Geometry check sheet. Reference: the model listing, model coordinates, mm. Round coordinates to 2 decimals unless told otherwise and drop trailing zeros. Order: outer loops, then holes, each group sorted by start corner. A loop starts at its lowest first (then second) coordinate and runs counter-clockwise, first axis right, second up.
```python
from build123d import *

# Parameters (mm, degrees)
F0_W          = 2.54
F0_H          = 2.54
F1_DEPTH      = 2.5
F2_SIZE       = 0.25
F3_W          = 0.7
F3_H          = 0.7
F4_DEPTH      = 2.7
F4_DEPTH_BACK = 8.9
F5_SIZE       = 0.1


with BuildPart() as f1:
    # F0 (on Top) → F1 (new body)
    with BuildSketch(Plane.XY):
        Rectangle(F0_W, F0_H)
    extrude(amount=F1_DEPTH)

    # F2
    f2_edges = [f1.edges().sort_by_distance(p)[0] for p in [
        (-1.27, -1.27, 1.25),
        (1.27, -1.27, 1.25),
        (1.27, 1.27, 1.25),
        (-1.27, 1.27, 1.25),
        (0, 1.27, 2.5),
        (1.27, 0, 2.5),
        (0, -1.27, 2.5),
        (-1.27, 0, 2.5),
        (1.27, 0, 0),
        (0, -1.27, 0),
        (-1.27, 0, 0),
        (0, 1.27, 0),
    ]]
    chamfer(f2_edges, length=F2_SIZE)

    # F3 (on face) → F4 (join, two sides)
    with BuildSketch(Plane.XY.offset(2.5)) as f4_sk:
        Rectangle(F3_W, F3_H)
    extrude(amount=F4_DEPTH)
    extrude(f4_sk.sketch, amount=-F4_DEPTH_BACK)

    # F5
    f5_edges = [f1.edges().sort_by_distance(p)[0] for p in [
        (0.35, 0, 5.2),
        (0, 0.35, 5.2),
        (-0.35, 0, 5.2),
        (0, -0.35, 5.2),
        (0.35, 0, -6.4),
        (0, -0.35, -6.4),
        (-0.35, 0, -6.4),
        (0, 0.35, -6.4),
    ]]
    chamfer(f5_edges, length=F5_SIZE)


solid = f1.part
```
(1) Depth check by flat-ended pin: P1, Ø0.8, axis at x = 0, z = -3, coming from the +Y side; P2, Ø0.8, axis at y = 0, z = 4, coming from the +X side; P3, Ø0.8, axis at y = 0, z = -4, coming from the -X side. Enter the tip coordinate at first touch or a pass-through.
Returned:
P1: stops at y = 0.35
P2: stops at x = 0.35
P3: stops at x = -0.35
(2) Sectioned sample at C-C, the plane z = 1.75. Record the cut outline in (x, y), and give its area (3 significant figures).
Returned:
outline: (-1.27, -1.02) - (-1.02, -1.27) - (1.02, -1.27) - (1.27, -1.02) - (1.27, 1.02) - (1.02, 1.27) - (-1.02, 1.27) - (-1.27, 1.02) - close
area: 6.33 mm2
(3) Sectioned sample at B-B, the plane x = -0.75. Record the cut outline in (y, z), and give its area (4 significant figures).
Returned:
outline: (-1.27, 0.25) - (-1.02, 0) - (1.02, 0) - (1.27, 0.25) - (1.27, 2.25) - (1.02, 2.5) - (-1.02, 2.5) - (-1.27, 2.25) - close
area: 6.225 mm2
(4) Sectioned sample at D-D, the plane z = -2.75. Record the cut outline in (x, y).
Returned:
outline: (-0.35, -0.35) - (0.35, -0.35) - (0.35, 0.35) - (-0.35, 0.35) - close
(5) Sectioned sample at A-A, the plane y = 0.15. Record the cut outline in (x, z), and give its area (3 significant figures).
Returned:
outline: (-1.27, 0.25) - (-1.02, 0) - (-0.35, 0) - (-0.35, -6.3) - (-0.25, -6.4) - (0.25, -6.4) - (0.35, -6.3) - (0.35, 0) - (1.02, 0) - (1.27, 0.25) - (1.27, 2.25) - (1.02, 2.5) - (0.35, 2.5) - (0.35, 5.1) - (0.25, 5.2) - (-0.25, 5.2) - (-0.35, 5.1) - (-0.35, 2.5) - (-1.02, 2.5) - (-1.27, 2.25) - close
area: 12.6 mm2
(6) Material ranges on line 1 (X direction, y = 0.05, z = 4); line 2 (Z direction, x = 0.5, y = -1), recorded low to high.
Returned:
line 1: x = -0.35 to 0.35
line 2: z = 0 to 2.5
